Input: dimensioned drawing with shaded views. Units: mm. Origin: part minimum x, y, z. A direction names the side the tool comes from. Round coordinates to 2 decimals unless told otherwise and drop trailing zeros. Loops run counter-clockwise (first coordinate to the right, second up) from the corner with the lowest first, then second, coordinate; pieces in that order, holes last. Notation, with made-up numbers: (-11.75, 69) - (41.25, 69) arc R12 cw to (41.25, 82) - close; hole circle Ø4 at (77, 37). An arc over 180 degrees is marked (long way). Answer as a JSON object with one key per item and string values. Group by question number.
Item 1: Draft query along X for the marked faces 3, 4 and 5. Return one class per face: released by +X, released by -X, zero draft, split by the parting line, or undercut.
Item 2: Section B-B (z = 27). Return the cut outline in (x, y), plus the area to 3 significant figures.
Item 3: Line query: line 1 (X direction, y = 2.5, z = 10); line 2 (X direction, y = 6.25, z = 58.5) (1 decimal); line 3 (Z direction, x = 120.5, y = 6.75). Output: solid intervals per line, ascending.
Item 4: Section C-C (x = 13). Return the cut outline in (y, z).
Item 5: Section D-D (y = 2). Count the separate pieces of the cut face and the enclosed holes in it, plus the area to 3 significant figures.
Item 6: Section A-A (x = 83). Return the cut outline in (y, z).
Item 7: Reachability of the marked faces 1 and 2 from +Z, -Z, +X, -X, +Y, -Y: full face, straight path, thin tool, end or side. Return the list, or none.
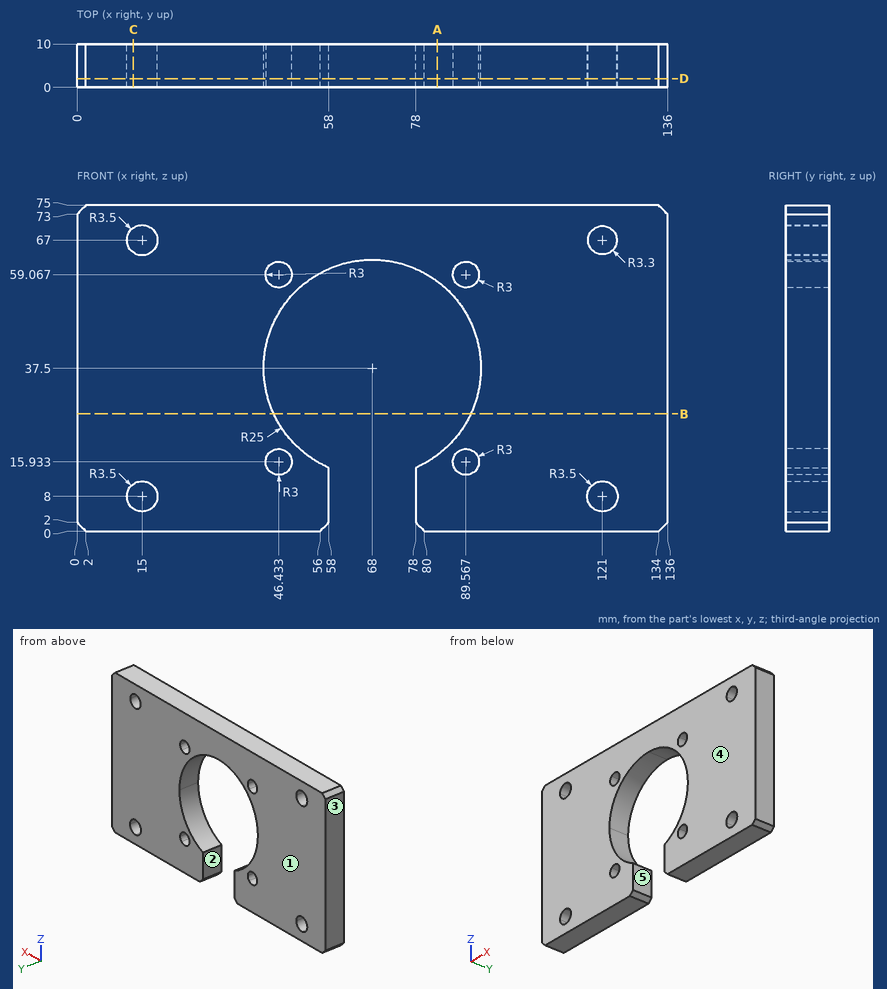
Values:
{
 "1": {"face 3": "released by -X", "face 4": "zero draft", "face 5": "undercut"},
 "2": {"outline": "(0, 0) - (45.31, 0) - (45.31, 10) - (0, 10) - close; (90.69, 0) - (136, 0) - (136, 10) - (90.69, 10) - close", "area": "906 mm^2"},
 "3": {"line 1": "x = 0 to 12.13, 17.87 to 58, 78 to 118.13, 123.87 to 136", "line 2": "x = 0 to 43.5, 49.4 to 54.4, 81.6 to 86.6, 92.5 to 136", "line 3": "z = 0 to 4.54, 11.46 to 63.74, 70.26 to 75"},
 "4": {"outline": "(0, 0) - (10, 0) - (10, 5.13) - (0, 5.13) - close; (0, 10.87) - (10, 10.87) - (10, 64.13) - (0, 64.13) - close; (0, 69.87) - (10, 69.87) - (10, 75) - (0, 75) - close"},
 "5": {"separate pieces": "1", "enclosed holes": "8", "area": "7,700 mm^2"},
 "6": {"outline": "(0, 0) - (10, 0) - (10, 17.5) - (0, 17.5) - close; (0, 57.5) - (10, 57.5) - (10, 75) - (0, 75) - close"},
 "7": {"face 1": "+Z, -Z, +X, -X, +Y", "face 2": "-Z, +Y, -Y"}
}
